Source: CAD feature listing. Evaluate the final solid. Frame: model axes, mm. Give positions to 0.01 mm unless a question says otherwise; leave off trailing zeros. Write each loop counter-clockwise with the first axis right and the second up, starting at its lowest first coordinate (ties: lowest second). Pieces come first, ordered by that corner, then holes. Notation, with made-up numbers: (-39, 35) -> (-20, 35) arc R31 ccw to (-20, 72) -> close; hole circle Ø5 at (58, -19.75). An arc over 180 degrees is marked (long way). Use one line per item in the form item = value. Start each with the question number.
(1) First-contact query: P1, Ø14.5, axis at x = -50, y = 0, coming from the +Z side; P2, Ø5.5, axis at x = 0, y = 50, coming from the -Z side; P3, Ø10, axis at x = 0, y = -50, coming from the +Z side. Flat tips, straight axial feed; report the tip coordinate or a pass-through.
(2) Material intervals for line 1 along Y through (x, z) = (0, 4); line 2 along Y through (x, z) = (-26.5, 14.5); line 3 along Y through (x, z) = (-50, 7), sorted ascending. Write a range as from..to.
(3) Cut plane B-B, the plane x = 50. Output: boundary loops of the cut face in (y, z) (3 decimals).
(4) Cut plane A-A, the plane z = 21.5. Count the separate pieces of the cut face and the enclosed holes in it, and give its area (3 significant figures).
from build123d import *

# Parameters (mm, degrees)
F0_W           = 130
F0_H           = 130
F1_DEPTH       = 27
F3_D           = 6.6
F3_CBORE_D     = 11.25
F3_CBORE_DEPTH = 15
F4_D           = 6.6
F4_DEPTH       = 15
F4_TIP         = 1.9828400428


with BuildPart() as f1:
    # F0 (on Top) → F1 (new body)
    with BuildSketch(Plane.XY):
        Rectangle(F0_W, F0_H)
    extrude(amount=F1_DEPTH)

    # F3 (through all)
    with Locations(Plane.XY.offset(27)):
        with Locations((0, 50), (-50, 0), (0, -50), (50, 0)):
            CounterBoreHole(F3_D / 2, F3_CBORE_D / 2, F3_CBORE_DEPTH)

    # F4
    with Locations(Plane.XY.offset(27)):
        with Locations((-25, 50), (-25, -50), (-50, -50), (-50, 50), (0, 0)):
            Hole(F4_D / 2, depth=F4_DEPTH)
            with Locations((0, 0, -(F4_DEPTH + F4_TIP / 2))):  # 118° drill point
                Cone(0, F4_D / 2, F4_TIP, mode=Mode.SUBTRACT)


solid = f1.part
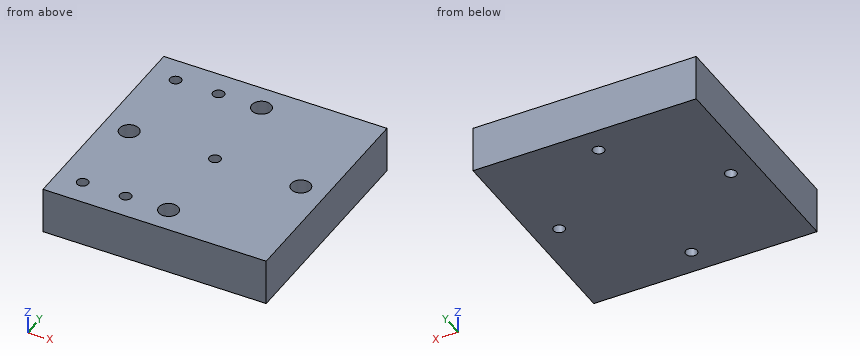
Geometry says:
q1.P1 = 27
q1.P2 = through
q1.P3 = 12
q2.line_1 = -65..-53.3, -46.7..46.7, 53.3..65
q2.line_2 = -65..-52.94, -47.06..47.06, 52.94..65
q2.line_3 = -65..-3.3, 3.3..65
q3.outline = (-65, 0) -> (-3.3, 0) -> (-3.3, 12) -> (-5.625, 12) -> (-5.625, 27) -> (-65, 27) -> close; (3.3, 0) -> (65, 0) -> (65, 27) -> (5.625, 27) -> (5.625, 12) -> (3.3, 12) -> close
q4.separate_pieces = 1
q4.enclosed_holes = 9
q4.area = 16,300 mm^2
